Work out the finished part from the listing and answer in its coordinate system (mm). Face numbers are marked on the shaded views. A direction names the side the tool comes from. Give positions to 0.01 mm unless a question says otherwise; leave off trailing zeros. Write each loop counter-clockwise with the first axis right and the second up, starting at its lowest first coordinate (ties: lowest second). Pieces come first, ordered by that corner, then holes. Notation, with made-up numbers: (18.5, -28.75) -> (77.5, -28.75) arc R12 cw to (77.5, -11.75) -> close; hole circle Ø8 at (84.25, 16). An arc over 180 degrees is marked (long way). Use a Markdown table: item, result. Add a question column.
Q1. Section D-D, the plane y = 31.5 is taken. Give the vertices of the cut face in (x, z), plus the area to 3 significant figures.
Q2. For the marked faces 1 and 2, determine the directions among +Z, -Z, +X, -X, +Y, -Y from which every point of the face is accessible in a straight line to the end or side of a thin tool.
Q3. Section B-B, the plane y = -10.5 is taken. Give the vertices of the cut face in (x, z).
Q4. Section C-C, the plane z = -24 is taken. Give the vertices of the cut face in (x, y), plus the area to 3 significant figures.
Q5. This flat-tipped pin is pushed along its axis until it touches: pin 1 Ø4 at (x, y) = (-26.5, 41.5) entering from +Z. Where does it stop, or does it pass through?
Q6. Section A-A, the plane x = -67 is taken. Give the vertices of the cut face in (y, z), plus the area to 3 significant figures.
Q7. Consider line 1 (Y direction, x = -30, z = -13); line 2 (X direction, y = -37.5, z = 25); line 3 (X direction, y = -48.5, z = 31.5). Determine where each line is inside the solid, lowest interval first.
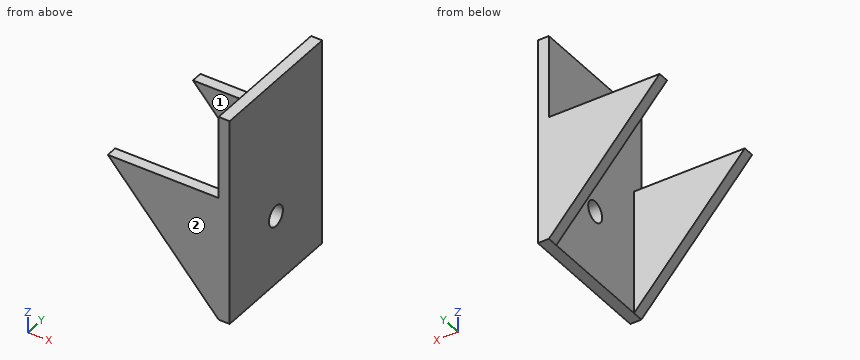
from build123d import *

# Parameters (mm, degrees)
F0_W     = 100
F0_H     = 150
F0_R     = 7.5
F1_DEPTH = 8
F2_W     = 8
F2_H     = 90
F3_DEPTH = 80
F5_DEPTH = 100.001


with BuildPart() as f1:
    # F0 (on Right) → F1 (new body)
    with BuildSketch(Plane.YZ):
        with Locations((-4.851894, 19.991098)):
            Rectangle(F0_W, F0_H)
        with Locations((-4.851894, -5.008902)):
            Circle(F0_R, mode=Mode.SUBTRACT)
    extrude(amount=F1_DEPTH)

    # F2 (on face) → F3 (join)
    with BuildSketch(Plane(origin=(0, 0, 0), x_dir=(0, -1, 0), z_dir=(-1, 0, 0))):
        with Locations((50.851894, -10.008902)):
            Rectangle(F2_W, F2_H)
        with Locations((-41.148106, -10.008902)):
            Rectangle(F2_W, F2_H)
    extrude(amount=F3_DEPTH)

    # F4 (on face) → F5 (cut, through all)
    with BuildSketch(Plane(origin=(0, 45.148106, 0), x_dir=(-1, 0, 0), z_dir=(0, 1, 0))):
        Polygon((80, -55.008902), (80, 34.991098), (0, -55.008902), align=None)
    extrude(amount=-F5_DEPTH, mode=Mode.SUBTRACT)


solid = f1.part
Result set:
| question | item | result |
|---|---|---|
| 1 | outline | (0, -55.01) -> (8, -55.01) -> (8, 94.99) -> (0, 94.99) -> close |
| 1 | area | 1,200 mm2 |
| 2 | face 1 | +Z, -Z, -X |
| 2 | face 2 | +Z, -Z, +X, -X, -Y |
| 3 | outline | (0, -55.01) -> (8, -55.01) -> (8, -9.94) -> (0, -9.94) -> close; (0, -0.07) -> (8, -0.07) -> (8, 94.99) -> (0, 94.99) -> close |
| 4 | outline | (-27.56, -54.85) -> (8, -54.85) -> (8, 45.15) -> (-27.56, 45.15) -> (-27.56, 37.15) -> (0, 37.15) -> (0, -46.85) -> (-27.56, -46.85) -> close |
| 4 | area | 1,240 mm2 |
| 5 | pin 1 | stops at z = 34.99 |
| 6 | outline | (-54.85, 20.37) -> (-46.85, 20.37) -> (-46.85, 34.99) -> (-54.85, 34.99) -> close; (37.15, 20.37) -> (45.15, 20.37) -> (45.15, 34.99) -> (37.15, 34.99) -> close |
| 6 | area | 234 mm2 |
| 7 | line 1 | y = -54.85 to -46.85, 37.15 to 45.15 |
| 7 | line 2 | x = 0 to 8 |
| 7 | line 3 | x = -76.9 to 8 |
